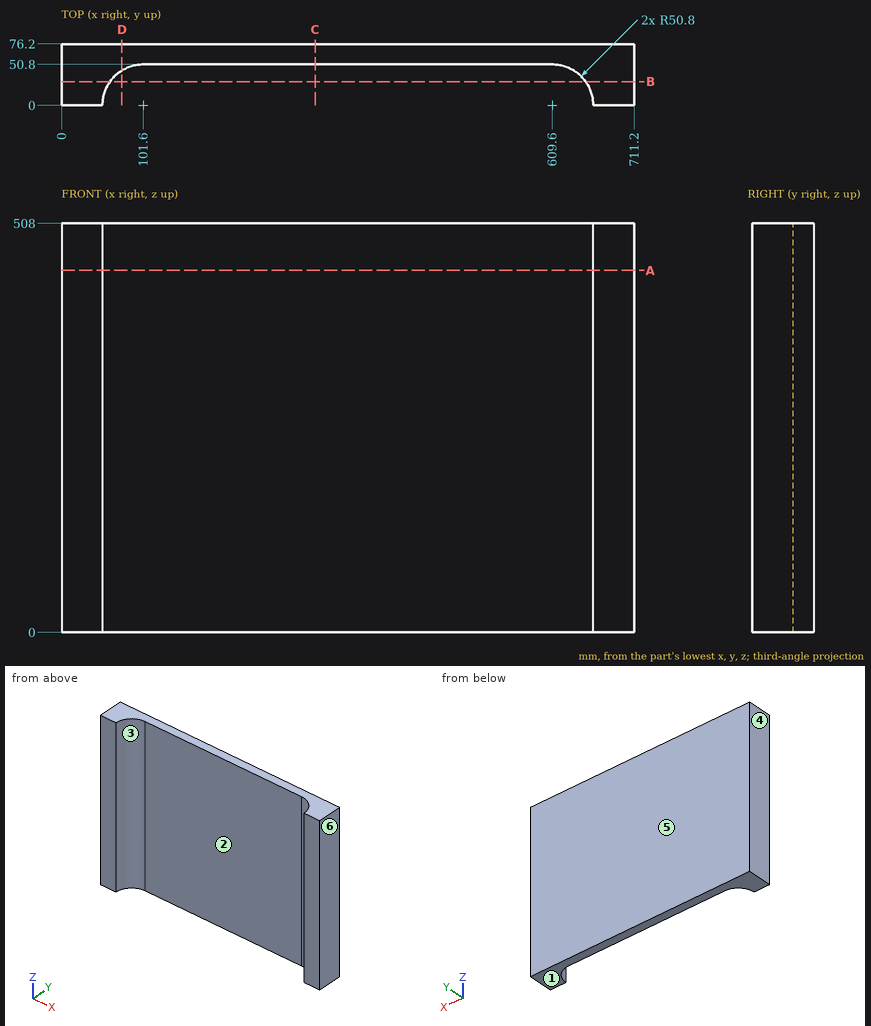
Can you work these out from the drawing? Everything is in mm from the part's minimum corner. A direction names the side the tool comes from. Round coordinates to 2 decimals unless told otherwise and drop trailing zeros. Order: outer loops, then holes, each group sorted by start corner. A loop starts at its lowest first (then second) coordinate and runs counter-clockwise, first axis right, second up. Notation, with made-up numbers: (66, -22.5) -> (98, -22.5) arc R27 cw to (98, 12.5) -> close; hole circle Ø11 at (62.25, 65). An arc over 180 degrees is marked (long way). Use CSV: the item, a comma, the result in double quotes.
1. Which directions (+Z, -Z, +X, -X, +Y, -Y) give clear straight access to the entire face, cutting with the end or side of a thin tool? Please do the marked faces 1 and 2.
Recorded:
face 1,"-Z, +X, -X, +Y, -Y"
face 2,"+Z, -Z, -Y"
2. I want a section at C-C on x = 315. List the corners of the cut face in (y, z) for me, and give its area (3 significant figures).
Recorded:
outline,"(50.8, 0) -> (76.2, 0) -> (76.2, 508) -> (50.8, 508) -> close"
area,"12,900 mm2"
3. I want a section at A-A on z = 449.5. List the corners of the cut face in (x, y) for me.
Recorded:
outline,"(0, 0) -> (50.8, 0) arc R50.8 cw to (101.6, 50.8) -> (609.6, 50.8) arc R50.8 cw to (660.4, 0) -> (711.2, 0) -> (711.2, 76.2) -> (0, 76.2) -> close"
4. I'm going to push a flat-ended pin straight in: P1, Ø1.5, axis at x = 361, z = 114, coming from the -Y side. Where does the tip first touch, or does it pass through?
Recorded:
P1,"stops at y = 50.8"
5. I need wall thicknesses on line 1 along Y through (x, z) = (548.5, 353.5); line 2 along X through (y, z) = (21.5, 399.5); line 3 along X through (y, z) = (27, 130). Which ranges of each line are inside material? Lowest first, please.
Recorded:
line 1,"y = 50.8 to 76.2"
line 2,"x = 0 to 55.57, 655.63 to 711.2"
line 3,"x = 0 to 58.57, 652.63 to 711.2"
6. Thinking about a two-plate mould opening in X: for the marked faces 3, 4, 5 and 6, which applies, pulls with the +X half, pulls with the -X half, needs draft (parallel to the pull), parting line crosses it, or undercut?
Recorded:
face 3,"undercut"
face 4,"pulls with the -X half"
face 5,"needs draft"
face 6,"pulls with the +X half"
7. I want a section at B-B on y = 29.5. List the corners of the cut face in (x, z) for me.
Recorded:
outline,"(0, 0) -> (60.24, 0) -> (60.24, 508) -> (0, 508) -> close; (650.96, 0) -> (711.2, 0) -> (711.2, 508) -> (650.96, 508) -> close"
8. I want a section at D-D on x = 75. List the corners of the cut face in (y, z) for me.
Recorded:
outline,"(43.28, 0) -> (76.2, 0) -> (76.2, 508) -> (43.28, 508) -> close"
